Here's the drawing with two shaded views (mm, measured from the low corner). I have some questions. A direction names the side the tool comes from. Coordinates: 2 decimals unless noted, no trailing zeros. Order: outer loops, then holes, each group sorted by start corner. A loop starts at its lowest first (then second) coordinate and runs counter-clockwise, first axis right, second up. Notation, with made-up numbers: (-1, 34.25) -> (24, 34.25) arc R27 ccw to (24, 56.25) -> close; hole circle Ø5 at (53, -31.5). An arc over 180 degrees is marked (long way). Answer as a JSON object with one key per item and string values. Group by question number.
(1) I want a section at C-C, the plane x = 22.5. List the corners of the cut face in (y, z) for me, plus the area to 3 significant figures.
(2) I want a section at D-D, the plane y = 13.5. List the corners of the cut face in (x, z) for me, plus the area to 3 significant figures.
(3) For pin 1 (4 mm diameter, centred on y = 7.5, z = 6.5, fed in from -X); pin 2 (2 mm diameter, centred on y = 2, z = 1.5, fed in from +X); pin 3 (2 mm diameter, centred on y = 9, z = 12, fed in from -X), each with a flat end and sliding along its axis, tell me the tip position at first contact or that it passes through.
(4) Which directions (+Z, -Z, +X, -X, +Y, -Y) give clear straight access to the entire face, cutting with the end or side of a thin tool? Please do the marked faces 5, 6 and 7.
(5) I want a section at A-A, the plane x = 13. List the corners of the cut face in (y, z) for me.
(6) I need wall thicknesses on line 1 (Y direction, x = 13, z = 6.75); line 2 (X direction, y = 2, z = 13); line 3 (X direction, y = 9, z = 9). Which ranges of each line are inside material? Lowest first, please.
(7) I want a section at B-B, the plane z = 13.75. List the corners of the cut face in (x, y) for me.
(8) If we mould it in two halves opening along Y, with no side actions, what happens to the marked faces 1, 2, 3 and 4? For each: pulls with the +Y half, pulls with the -Y half, needs draft (parallel to the pull), parting line crosses it, or undercut.
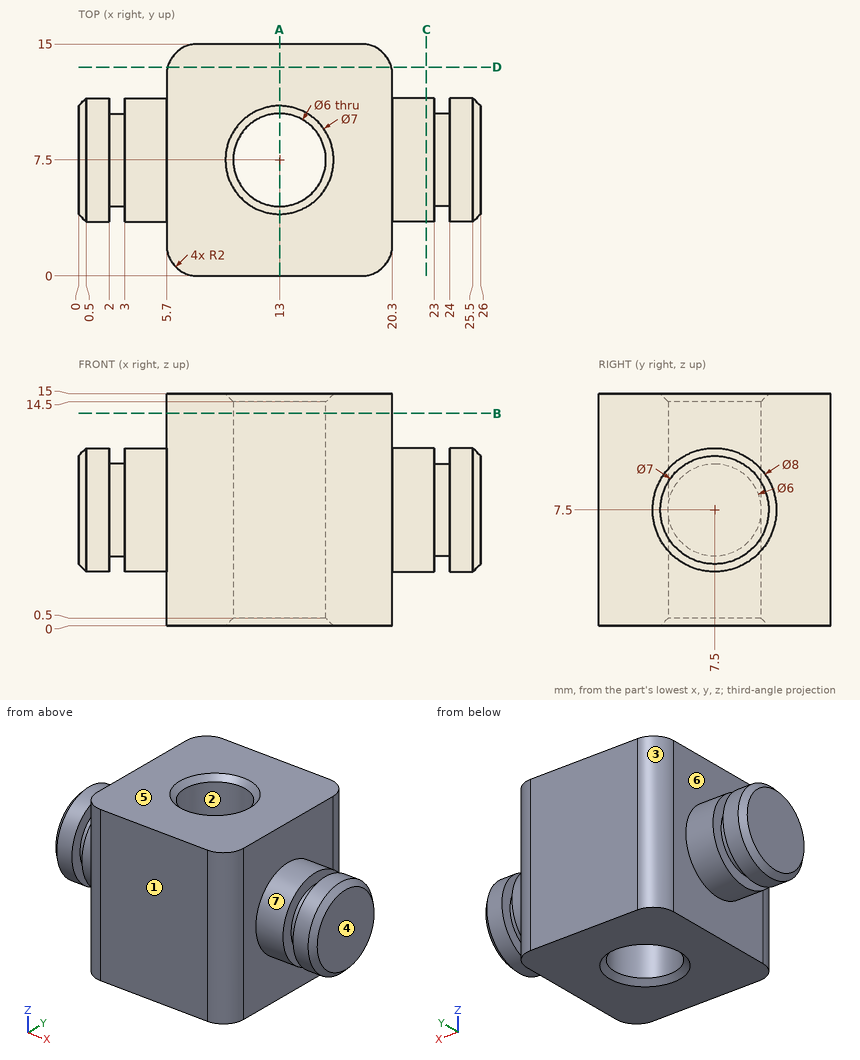
Computed values:
{
 "1": {"outline": "circle Ø8 at (7.5, 7.5)", "area": "50.3 mm2"},
 "2": {"outline": "(5.76, 0) -> (20.24, 0) -> (20.24, 15) -> (5.76, 15) -> close", "area": "217 mm2"},
 "3": {"pin 1": "stops at x = 0", "pin 2": "stops at x = 20.3", "pin 3": "stops at x = 0.24"},
 "4": {"face 5": "+Z, +X, -X, +Y, -Y", "face 6": "-X", "face 7": "+X"},
 "5": {"outline": "(0, 0) -> (4, 0) -> (4.5, 0.5) -> (4.5, 14.5) -> (4, 15) -> (0, 15) -> close; (10.5, 0.5) -> (11, 0) -> (15, 0) -> (15, 15) -> (11, 15) -> (10.5, 14.5) -> close"},
 "6": {"line 1": "y = 0 to 4.5, 10.5 to 15", "line 2": "x = 5.7 to 20.3", "line 3": "x = 0 to 10.4, 15.6 to 26"},
 "7": {"outline": "(5.7, 2) arc R2 ccw to (7.7, 0) -> (18.3, 0) arc R2 ccw to (20.3, 2) -> (20.3, 13) arc R2 ccw to (18.3, 15) -> (7.7, 15) arc R2 ccw to (5.7, 13) -> close; hole circle Ø6 at (13, 7.5)"},
 "8": {"face 1": "pulls with the -Y half", "face 2": "undercut", "face 3": "pulls with the +Y half", "face 4": "needs draft"}
}
